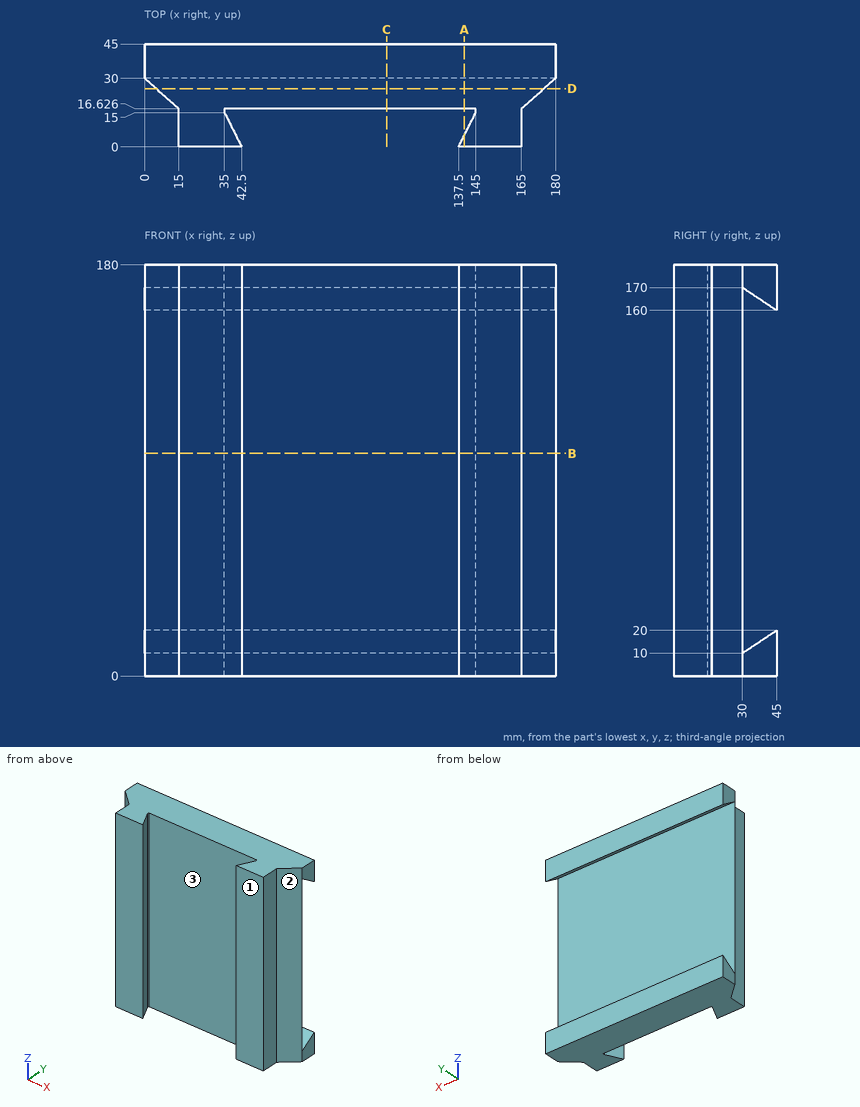
Geometry check sheet. Reference: drawing and pictorial views, mm from the part's lowest x, y, z. Coordinates: 2 decimals unless noted, no trailing zeros. Write each loop counter-clockwise with the first axis right and the second up, starting at its lowest first coordinate (ties: lowest second). Pieces come first, ordered by that corner, then holes. Notation, with made-up numbers: (-23.75, -15.75) - (9.25, -15.75) arc R10 cw to (9.25, 0.25) - close; hole circle Ø9 at (34, 8). An arc over 180 degrees is marked (long way). One line per question, with ' | ' between items. Start each with the question number.
1. Section check A-A (x = 140). Enter the section's corners in (y, z), plus the area to 3 significant figures.
2. Draft check along X on the marked faces 1, 2 and 3. Enter one of: released by +X, released by -X, zero draft, split by the parting line, or undercut.
3. Section check D-D (y = 25.5). Enter the section's corners in (x, z), plus the area to 3 significant figures.
4. Section check B-B (z = 97.5). Enter the section's corners in (x, y), plus the area to 3 significant figures.
5. Section check C-C (x = 106). Enter the section's corners in (y, z).
6. Gauge pin test, flat ends, axial feed: P1, Ø0.5, axis at y = 16, z = 102.5, coming from the -X side; P2, Ø12, axis at y = 22, z = 110.5, coming from the -X side; P3, Ø12, axis at y = 34.5, z = 155.5, coming from the +X side. Record the tip position at first contact, or that the pin passes through.
7. Material ranges on line 1 along Y through (x, z) = (142.5, 76) (1 decimal); line 2 along Y through (x, z) = (21, 96); line 3 along X through (y, z) = (16, 151), recorded low to high.
Computed values:
1) outline: (0, 0) - (5, 0) - (5, 180) - (0, 180) - close; (16.63, 0) - (45, 0) - (45, 20) - (30, 10) - (30, 170) - (45, 160) - (45, 180) - (16.63, 180) - close | area: 3,760 mm²
2) face 1: zero draft | face 2: released by +X | face 3: undercut
3) outline: (5.05, 0) - (174.95, 0) - (174.95, 180) - (5.05, 180) - close | area: 30,600 mm²
4) outline: (0, 30) - (15, 16.63) - (15, 0) - (42.5, 0) - (35, 15) - (35, 16.63) - (145, 16.63) - (145, 15) - (137.5, 0) - (165, 0) - (165, 16.63) - (180, 30) - close | area: 2,980 mm²
5) outline: (16.63, 0) - (45, 0) - (45, 20) - (30, 10) - (30, 170) - (45, 160) - (45, 180) - (16.63, 180) - close
6) P1: x = 15 | P2: x = 2.24 | P3: x = 180
7) line 1: 0 to 10, 16.6 to 30 | line 2: 0 to 30 | line 3: 15 to 35, 145 to 165
